Can you work these out from the model? Positions are in its coordinate system, mm. Coordinates: 2 decimals unless noted, no trailing zeros. Order: outer loops, then holes, each group sorted by start corner. A loop starts at its lowest first (then second) coordinate and runs counter-clockwise, first axis right, second up. Notation, with made-up numbers: (75.5, -23) -> (85.5, -23) arc R27 cw to (85.5, 10) -> close; hole circle Ø2 at (76, -28). An arc over 180 degrees is marked (long way). Write item = value, one per line. Start each with the question number.
from build123d import *

# Parameters (mm, degrees)
SKETCH1_W                                         = 63.5
SKETCH1_H                                         = 12.7
BOSS_EXTRUDE1_DEPTH                               = 101.6
FILLET1_R                                         = 12.7
CSK_FOR_8_FLAT_HEAD_MACHINE_SCREW_100_D           = 4.4958
CSK_FOR_8_FLAT_HEAD_MACHINE_SCREW_100_CSINK_D     = 8.4328
CSK_FOR_8_FLAT_HEAD_MACHINE_SCREW_100_CSINK_ANGLE = 100
FILLET2_R                                         = 1.5875


with BuildPart() as part:
    # Sketch1 → Boss-Extrude1 (new, symmetric)
    with BuildSketch(Plane.XY):
        Rectangle(SKETCH1_W, SKETCH1_H)
    extrude(amount=BOSS_EXTRUDE1_DEPTH, both=True)

    # Fillet1
    fillet1_edges = [part.edges().sort_by_distance(p)[0] for p in [
        (-31.75, 0, 101.6),
        (31.75, 0, 101.6),
        (-31.75, 0, -101.6),
        (31.75, 0, -101.6),
    ]]
    fillet(fillet1_edges, radius=FILLET1_R)

    # CSK for #8 Flat Head Machine Screw (100)1 (through all)
    with Locations(Plane(origin=(0, 6.35, 0), x_dir=(1, 0, 0), z_dir=(0, 1, 0))):
        with Locations((19.05, -88.9), (-19.05, -88.9), (-19.05, 88.9), (19.05, 88.9), (0, -38.1), (0, 38.1), (0, 0)):
            CounterSinkHole(CSK_FOR_8_FLAT_HEAD_MACHINE_SCREW_100_D / 2, CSK_FOR_8_FLAT_HEAD_MACHINE_SCREW_100_CSINK_D / 2, counter_sink_angle=CSK_FOR_8_FLAT_HEAD_MACHINE_SCREW_100_CSINK_ANGLE)

    # Fillet2
    fillet2_edges = [part.edges().sort_by_distance(p)[0] for p in [
        (-31.75, 6.35, 0),
        (0, 6.35, -101.6),
        (0, 6.35, 101.6),
        (31.75, 6.35, 0),
        (28.030256121, 6.35, 97.880256121),
        (-28.030256121, 6.35, 97.880256121),
        (28.030256121, 6.35, -97.880256121),
        (-28.030256121, 6.35, -97.880256121),
    ]]
    fillet(fillet2_edges, radius=FILLET2_R)


solid = part.part
(1) Thinking about a two-plate mould opening in Z: for faces 1 (the face through (-7, 6.35, 1)), 2 (the face through (27.93, -0.72, 97.98)), 3 (the face through (20.8, 4.8, -90.5)), which applies, +Z half, -Z half, draft (parallel to the pull), parting line (faces both ways), or undercut?
(2) Imagine slicing it at A-A (y = -0.5). Write out the boundary of the cut face in (x, z).
(3) For P1, Ø5, axis at x = 19.05, z = -88.9, coming from the +Y side; P2, Ø3.5, axis at x = 19.05, z = 88.9, coming from the +Y side; P3, Ø7, axis at x = 0, z = 0, coming from the +Y side; P4, Ø6, axis at x = 0, z = 38.1, coming from the +Y side, each with a flat end and sliding along its axis, tell me the tip position at first contact or that it passes through.
(4) If I drill on L1, parallel to Z at x = -19.05, y = -3; L2, parallel to Z at x = 0, y = 0.25; L3, parallel to X at y = -3.25, z = -88.9, over which ranges is the centre line in solid material (lowest first)? Write a range as from..to.
Result set:
q1.face_1 = draft
q1.face_2 = +Z half
q1.face_3 = undercut
q2.outline = (-31.75, -88.9) arc R12.7 ccw to (-19.05, -101.6) -> (19.05, -101.6) arc R12.7 ccw to (31.75, -88.9) -> (31.75, 88.9) arc R12.7 ccw to (19.05, 101.6) -> (-19.05, 101.6) arc R12.7 ccw to (-31.75, 88.9) -> close; hole circle Ø4.5 at (-19.05, -88.9); hole circle Ø4.5 at (-19.05, 88.9); hole circle Ø4.5 at (0, -38.1); hole circle Ø4.5 at (0, 0); hole circle Ø4.5 at (0, 38.1); hole circle Ø4.5 at (19.05, -88.9); hole circle Ø4.5 at (19.05, 88.9)
q3.P1 = 4.91
q3.P2 = through
q3.P3 = 5.75
q3.P4 = 5.33
q4.L1 = -101.6..-91.15, -86.65..86.65, 91.15..101.6
q4.L2 = -101.6..-40.35, -35.85..-2.25, 2.25..35.85, 40.35..101.6
q4.L3 = -31.75..-21.3, -16.8..16.8, 21.3..31.75
